Autodesk Inventor part; units mm, degrees
ref_plane "Work Plane2" through (-220.8757, 0, -44.2597) normal (-0.9238795, 0, -0.3826834) x (0, 1, 0)
ref_plane "Work Plane4" through (-216.1663, 15, -57.9216) normal (0.9238795, 0, 0.3826834) x (0, -1, 0)
ref_plane "YZ Plane" through (0, 0, 0) normal (1, 0, 0) x (0, 1, 0)
sketch "Sketch1" plane through (0, 0, 0) normal (0, 1, 0) x (-1, 0, 0)
  circle A0 centre (0, 0) radius 217.5
  circle A1 centre (0, 0) radius 312.5
  line L0 (0, 0) -> (220.9709, -220.9709)
  line L1 (0, 0) -> (312.5, 0) construction
  line L2 (312.1398, -15) -> (216.9821, -15)
  line L3 (231.3228, -210.1096) -> (164.0361, -142.8229)
  circle A2 centre (0, 0) radius 240
  circle A3 centre (0, 0) radius 290
  line L4 (285.6571, -50) -> (234.7339, -50)
  line L5 (237.3454, -166.6348) -> (201.3373, -130.6266)
  dimension "d0" = 435
  dimension "d1" = 625
  dimension "d2" = 45
  dimension "d3" = 15
  dimension "d4" = 15
  dimension "d5" = 22.5
  dimension "d6" = 22.5
  dimension "d7" = 35
  dimension "d8" = 35
extrude "Extrusion1" add sketch "Sketch1" along normal blind 10 contours A2 L4 A3 L5
sketch "Sketch2" plane through (0, 10, 0) normal (0, 1, 0) x (1, 0, 0)
  arc A0 (-237.3454, 166.6348) -> (-285.6571, 50) centre (0, 0) ccw
  line L0 (-285.6571, 50) -> (-234.7339, 50)
  arc A1 (-201.3373, 130.6266) -> (-234.7339, 50) centre (0, 0) ccw
  line L1 (-201.3373, 130.6266) -> (-237.3454, 166.6348)
  circle A2 centre (0, 0) radius 245
  circle A3 centre (0, 0) radius 285
  line L2 (-279.6426, 55) -> (-238.7467, 55)
  line L3 (-236.6281, 158.8463) -> (-207.7103, 129.9286)
  line L4 (-239.8437, 50) -> (-280.5798, 50)
  line L5 (-204.9504, 134.2398) -> (-233.7552, 163.0445)
  dimension "d11" = 5
  dimension "d12" = 5
  dimension "d13" = 5
  dimension "d14" = 5
extrude "Extrusion2" cut sketch "Sketch2" against normal up to surface (10 mm away) contours L3 A2 L2 A3
sketch "Sketch3" plane through (0, 10, 0) normal (0, 1, 0) x (1, 0, 0)
  arc A0 (-236.6281, 158.8463) -> (-279.6426, 55) centre (0, 0) ccw
  line L0 (-236.6281, 158.8463) -> (-207.7103, 129.9286)
  arc A1 (-207.7103, 129.9286) -> (-238.7467, 55) centre (0, 0) ccw
  line L1 (-238.7467, 55) -> (-279.6426, 55)
  arc A2 (-237.3454, 166.6348) -> (-285.6571, 50) centre (0, 0) ccw
  line L2 (-285.6571, 50) -> (-234.7339, 50)
  arc A3 (-201.3373, 130.6266) -> (-234.7339, 50) centre (0, 0) ccw
  line L3 (-201.3373, 130.6266) -> (-237.3454, 166.6348)
  circle A4 centre (0, 0) radius 217.5
  circle A5 centre (0, 0) radius 312.5
  line L4 (0, 0) -> (100, 0) construction
  line L5 (0, 0) -> (-220.9709, 220.9709)
  line L6 (0, 0) -> (312.5, 0) construction
  line L7 (-312.1398, 15) -> (-216.9821, 15)
  line L8 (-164.0361, 142.8229) -> (-231.3228, 210.1096)
  line L9 (-437.5, 0) -> (437.5, 0)
  dimension "d17" = 435
  dimension "d18" = 625
  dimension "d21" = 135
  dimension "d22" = 15
  dimension "d23" = 15
extrude "Extrusion3" add sketch "Sketch3" along normal blind 5 contours L0 A1 L1 A0 | L3 A3 L2 A2 | A4 L7 A5 L8
sketch "Sketch4" plane through (0, 15, 0) normal (0, 1, 0) x (1, 0, 0)
  arc A0 (-231.3228, 210.1096) -> (-312.1398, 15) centre (0, 0) ccw
  line L0 (-312.1398, 15) -> (-216.9821, 15)
  arc A1 (-164.0361, 142.8229) -> (-216.9821, 15) centre (0, 0) ccw
  line L1 (-164.0361, 142.8229) -> (-231.3228, 210.1096)
  circle A2 centre (0, 0) radius 217.5
  circle A3 centre (0, 0) radius 312.5
  line L2 (0, 0) -> (4.6194, -1.9134) construction
  line L3 (0, 0) -> (5, 0) construction
  circle A4 centre (4.6194, -1.9134) radius 242.5
  circle A5 centre (4.6194, -1.9134) radius 297.5
  line L4 (0, 0) -> (-288.7124, 119.5886) construction
  line L5 (0, 0) -> (-270.6329, 156.25)
  line L6 (0, 0) -> (-301.8518, 80.881)
  circle A6 centre (4.6194, -1.9134) radius 228.75
  circle A7 centre (4.6194, -1.9134) radius 311.25
  point P0 (-253.3489, 146.271)
  point P1 (-217.3642, 196.151)
  point P2 (-282.5739, 75.7155)
  point P3 (-292.3994, 15)
  point P4 (-205.7173, 118.7709)
  point P5 (-188.3605, 108.75)
  point P6 (-178.396, 157.1828)
  point P7 (-210.0889, 56.2931)
  point P8 (-229.4479, 61.4804)
  point P9 (-237.2901, 15)
  point P10 (-295.8554, 79.2742)
  point P11 (-265.2567, 153.146)
  point P12 (-193.8094, 111.8959)
  point P13 (-216.1663, 57.9216)
  dimension "d26" = 625
  dimension "d27" = 435
  dimension "d28" = 5
  dimension "d29" = 22.5
  dimension "d30" = 485
  dimension "d31" = 595
  dimension "d33" = 15
  dimension "d36" = 457.5
  dimension "d37" = 622.5
extrude "Extrusion4" cut sketch "Sketch4" against normal blind 10 contours L1 A7 L5 A0 | L5 A7 L6 A0 | L1 A5 L5 A7 | L6 A7 L0 A0 | L6 A5 L0 A7 | L1 A6 L5 A4 | L1 A1 L5 A6 | L6 A6 L0 A4 | L5 A1 L6 A6 | L6 A1 L0 A6
sketch "Sketch5" plane through (0, 15, 0) normal (0, 1, 0) x (1, 0, 0)
  arc A0 (-282.5739, 75.7155) -> (-292.3994, 15) centre (4.6194, -1.9134) ccw
  line L0 (-292.3994, 15) -> (-237.2901, 15)
  arc A1 (-229.4479, 61.4804) -> (-237.2901, 15) centre (4.6194, -1.9134) ccw
  line L1 (-229.4479, 61.4804) -> (-216.1663, 57.9216)
  arc A2 (-193.8094, 111.8959) -> (-216.1663, 57.9216) centre (4.6194, -1.9134) ccw
  line L2 (-193.8094, 111.8959) -> (-205.7173, 118.7709)
  arc A3 (-178.396, 157.1828) -> (-205.7173, 118.7709) centre (4.6194, -1.9134) ccw
  line L3 (-178.396, 157.1828) -> (-217.3642, 196.151)
  arc A4 (-217.3642, 196.151) -> (-253.3489, 146.271) centre (4.6194, -1.9134) ccw
  line L4 (-253.3489, 146.271) -> (-265.2567, 153.146)
  arc A5 (-265.2567, 153.146) -> (-295.8554, 79.2742) centre (4.6194, -1.9134) ccw
  line L5 (-295.8554, 79.2742) -> (-282.5739, 75.7155)
  arc A6 (-157.7572, 146.5246) -> (-215.1597, 7.9427) centre (4.6194, -1.9134) ccw
  arc A7 (-254.0861, 186.4253) -> (-311.4886, 47.8434) centre (4.6194, -1.9134) ccw
  line L6 (-311.4886, 47.8434) -> (-215.1597, 7.9427)
  line L7 (-157.7572, 146.5246) -> (-254.0861, 186.4253)
  line L8 (-291.0221, 120.5453) -> (-198.6341, 82.2769) construction
  line L9 (-282.9381, 117.1968) -> (-206.718, 85.6254) construction
  point P0 (0, 0)
  point P1 (-244.8281, 101.4111)
  point P2 (-244.8281, 101.4111)
  point P3 (-232.656, 177.5487)
  point P4 (-179.7358, 155.6284)
  point P5 (-237.1383, 17.0465)
  point P6 (-290.0585, 38.9667)
  dimension "d38" = 150
  dimension "d39" = 104.2656
extrude "Extrusion5" cut sketch "Sketch5" against normal blind 10 contours L6 A1 L0 A0 | A4 L3 A3 L7
ref_plane "Work Plane2" through (-220.8757, 0, -44.2597) normal (-0.9238795, 0, -0.3826834) x (0, 1, 0)
ref_plane "Work Plane1" through (-234.7339, 0, -50) normal (-0.9238795, 0, -0.3826834) x (0, 1, 0)
sketch "Sketch7" plane through (0, 10, 0) normal (0, -1, 0) x (1, 0, 0)
  arc A0 (-279.6426, -55) -> (-236.6281, -158.8463) centre (0, 0) ccw
  line L0 (-236.6281, -158.8463) -> (-207.7103, -129.9286)
  arc A1 (-238.7467, -55) -> (-207.7103, -129.9286) centre (0, 0) ccw
  arc A2 (-238.7467, -55) -> (-207.7103, -129.9286) centre (0, 0) ccw
  line L1 (-238.7467, -55) -> (-279.6426, -55)
  arc A3 (-279.6426, -55) -> (-236.6281, -158.8463) centre (0, 0) ccw
  arc A4 (-291.5761, -93.715) -> (-272.4419, -139.9089) centre (4.6194, 1.9134) ccw
  line L2 (-195.885, -108.198) -> (-272.4419, -139.9089)
  arc A5 (-215.0192, -62.0041) -> (-195.885, -108.198) centre (4.6194, 1.9134) ccw
  line L3 (-215.0192, -62.0041) -> (-291.5761, -93.715)
  arc A6 (-279.6426, -55) -> (-236.6281, -158.8463) centre (0, 0) ccw
  line L4 (-279.6426, -55) -> (-238.7467, -55)
  arc A7 (-238.7467, -55) -> (-207.7103, -129.9286) centre (0, 0) ccw
  line L5 (-207.7103, -129.9286) -> (-236.6281, -158.8463)
  arc A8 (-285.6571, -50) -> (-237.3454, -166.6348) centre (0, 0) ccw
  line L6 (-201.3373, -130.6266) -> (-237.3454, -166.6348)
  arc A9 (-234.7339, -50) -> (-201.3373, -130.6266) centre (0, 0) ccw
  line L7 (-285.6571, -50) -> (-234.7339, -50)
  line L8 (-233.2223, -155.4405) -> (-236.0507, -152.6121) construction
  line L9 (-236.0507, -152.6121) -> (-238.8791, -155.4405) construction
  line L10 (-209.8621, -132.0804) -> (-212.6905, -129.2519) construction
  line L11 (-212.6905, -129.2519) -> (-209.8621, -126.4235) construction
  circle A10 centre (-212.6905, -129.2519) radius 1.75
  circle A11 centre (-236.0507, -152.6121) radius 1.75
  line L12 (-274.8261, -55) -> (-274.8261, -59) construction
  line L13 (-274.8261, -59) -> (-278.8261, -59) construction
  line L14 (-241.7898, -55) -> (-241.7898, -59) construction
  line L15 (-241.7898, -59) -> (-237.7898, -59) construction
  circle A12 centre (-241.7898, -59) radius 1.75
  circle A13 centre (-274.8261, -59) radius 1.75
  line L16 (-233.2223, -162.5116) -> (-226.8583, -156.1476)
  line L17 (-226.8583, -156.1476) -> (-236.0507, -146.9553)
  line L18 (-236.0507, -146.9553) -> (-242.4147, -153.3192)
  line L19 (-242.4147, -153.3192) -> (-233.2223, -162.5116)
  line L20 (-209.155, -138.4443) -> (-201.3373, -130.6266)
  line L21 (-201.3373, -130.6266) -> (-210.5297, -121.4342)
  line L22 (-210.5297, -121.4342) -> (-218.3474, -129.2519)
  line L23 (-218.3474, -129.2519) -> (-209.155, -138.4443)
  line L24 (-285.6571, -50) -> (-270.8261, -50)
  line L25 (-270.8261, -50) -> (-270.8261, -63)
  line L26 (-270.8261, -63) -> (-285.6571, -63)
  line L27 (-285.6571, -63) -> (-285.6571, -50)
  line L28 (-234.7339, -50) -> (-245.7898, -50)
  line L29 (-245.7898, -50) -> (-245.7898, -63)
  line L30 (-245.7898, -63) -> (-234.7339, -63)
  line L31 (-234.7339, -63) -> (-234.7339, -50)
  line L32 (-236.6281, -158.8463) -> (-207.7103, -129.9286)
  line L33 (-238.7467, -55) -> (-279.6426, -55)
  arc A14 (-279.6426, -55) -> (-236.6281, -158.8463) centre (0, 0) ccw
  line L34 (-236.6281, -158.8463) -> (-207.7103, -129.9286)
  arc A15 (-238.7467, -55) -> (-207.7103, -129.9286) centre (0, 0) ccw
  line L35 (-238.7467, -55) -> (-279.6426, -55)
  point P0 (-214.4385, -125.3431)
  point P1 (-277.9496, -63)
  point P2 (-270.8261, -55)
  point P3 (-236.7615, -63)
  point P4 (-245.7898, -55)
  point P5 (-212.6905, -134.9088)
  point P6 (-211.9634, -122.8679)
  point P7 (-241.0878, -151.9923)
  point P8 (-230.3939, -152.6121)
  dimension "d51" = 4
  dimension "d52" = 4
  dimension "d54" = 4
  dimension "d55" = 4
  dimension "d56" = 3.5
  dimension "d57" = 3.5
  dimension "d58" = 4
  dimension "d59" = 4
  dimension "d60" = 4
  dimension "d61" = 4
  dimension "d62" = 3.5
  dimension "d63" = 3.5
  dimension "d64" = 4
  dimension "d65" = 4
  dimension "d66" = 5
  dimension "d71" = 4
  dimension "d72" = 4
  dimension "d73" = 4
  dimension "d74" = 4
  dimension "d75" = 4
  dimension "d76" = 4
extrude "Extrusion7" add sketch "Sketch7" along normal blind 10 contours L1 L25 L26 A0 | L1 A1 L30 L29 | L18 L17 L0 A0 | A1 L0 L23 L22
extrude "Extrusion8" cut sketch "Sketch7" against normal up to next contours A10 | A11 | A12 | A13
ref_plane "Work Plane4" through (-216.1663, 15, -57.9216) normal (0.9238795, 0, 0.3826834) x (0, -1, 0)
sketch "Sketch9" plane through (-216.1663, 15, -57.9216) normal (0.9238795, 0, 0.3826834) x (0, -1, 0)
  line L0 (5, 58.4214) -> (5, 0)
  line L1 (0, 58.4214) -> (5, 58.4214)
  line L2 (0, 0) -> (0, 58.4214)
  line L3 (0, 0) -> (5, 0)
  line L4 (15, -14.4241) -> (15, 72.8455)
  line L5 (15, 72.8455) -> (5, 72.8455)
  line L6 (5, -14.4241) -> (5, 72.8455)
  line L7 (15, -14.4241) -> (5, -14.4241)
  line L8 (-2, 5.2107) -> (2, 5.2107)
  line L9 (2, 5.2107) -> (2, 53.2107)
  line L10 (2, 53.2107) -> (-2, 53.2107)
  line L11 (-2, 53.2107) -> (-2, 5.2107)
  line L12 (-2, 5.2107) -> (2, 53.2107) construction
  line L13 (2, 5.2107) -> (-2, 53.2107) construction
  point P0 (15, 29.2107)
  point P1 (0, 29.2107)
  dimension "d85" = 4
  dimension "d86" = 48
extrude "Extrusion10" cut sketch "Sketch9" against normal up to next contours L10 L9 L8 L2 | L2 L8 L11 L10
sketch "Sketch10" plane through (0, 10, 0) normal (0, -1, 0) x (1, 0, 0)
  arc A0 (-291.2664, -94.6691) -> (-272.8976, -139.0153) centre (4.6194, 1.9134) ccw
  line L0 (-214.736, -62.9692) -> (-291.2664, -94.6691)
  arc A1 (-214.736, -62.9692) -> (-196.3672, -107.3154) centre (4.6194, 1.9134) ccw
  line L1 (-196.3672, -107.3154) -> (-272.8976, -139.0153)
  line L2 (-245.7898, -63) -> (-245.7898, -55)
  line L3 (-245.7898, -55) -> (-270.8261, -55)
  line L4 (-270.8261, -55) -> (-270.8261, -63)
  line L5 (-270.8261, -63) -> (-277.9496, -63)
  arc A2 (-277.9496, -63) -> (-241.0878, -151.9923) centre (0, 0) ccw
  line L6 (-241.0878, -151.9923) -> (-236.0507, -146.9553)
  line L7 (-236.0507, -146.9553) -> (-230.3939, -152.6121)
  line L8 (-230.3939, -152.6121) -> (-212.6905, -134.9088)
  line L9 (-212.6905, -134.9088) -> (-218.3474, -129.2519)
  line L10 (-218.3474, -129.2519) -> (-211.9634, -122.8679)
  arc A3 (-236.7615, -63) -> (-211.9634, -122.8679) centre (0, 0) ccw
  line L11 (-236.7615, -63) -> (-245.7898, -63)
  point P0 (-216.0774, -115.4796)
  point P1 (-234.4462, -71.1334)
  point P2 (-271.5548, -86.5043)
  point P3 (-253.186, -130.8505)
extrude "Extrusion11" cut sketch "Sketch10" against normal blind 10 contours L0 A3 L1 A2
properties part number "Battery Module Third Iteration Top wING" material "PLA Plastic"
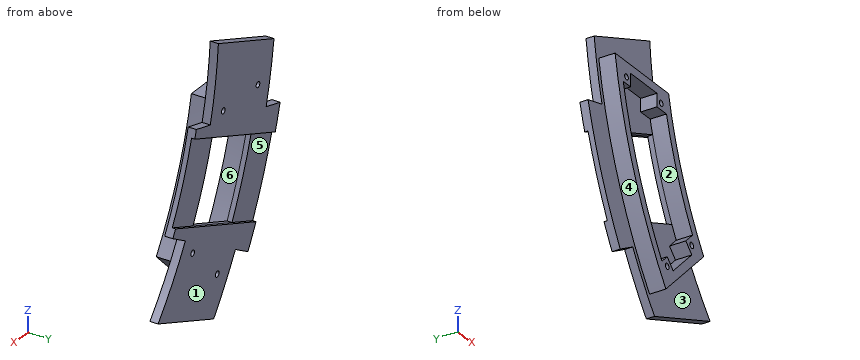
Geometry: final body of the model. Coordinates: model frame, mm. Face numbers are marked on the shaded views. A direction names the side the tool comes from. Give positions to 0.01 mm unless a question says otherwise; leave off trailing zeros. Write each loop counter-clockwise with the first axis right and the second up, starting at its lowest first coordinate (ties: lowest second). Pieces come first, ordered by that corner, then holes. Notation, with made-up numbers: (-21, 4.5) -> (15, 4.5) arc R17 cw to (15, 19.5) -> close; hole circle Ø6 at (51.5, 15.5). An arc over 180 degrees is marked (long way). Answer in a Markdown table with one row per item.
(1) Section query C-C on z = -69. Return loops of the section in (x, y), then the cut area to 3 significant figures.
Answers below:
| item | result |
|---|---|
| outline | (-284.31, 10) -> (-281.67, 10) -> (-281.67, 0) -> (-276.52, 0) -> (-276.52, 10) -> (-235.08, 10) -> (-235.08, 0) -> (-229.87, 0) -> (-229.87, 10) -> (-212.86, 10) -> (-212.86, 13) -> (-229.3, 13) -> (-229.3, 15) -> (-284.31, 15) -> close |
| area | 428 mm^2 |
(2) Set-up query: the marked faces 1 and 2. Return all of +Z, -Z, +X, -X, +Y, -Y with unobstructed straight access to the full face (end or side cutting, diameter ignored); none if empty.
Answers below:
| item | result |
|---|---|
| face 1 | +Z, -Z, +X, -X, +Y |
| face 2 | -Y |
(3) Pin query (flat end, axial travel): pin 1 (4 mm diameter, centred on y = 1.5, z = -118.5, fed in from +X); pin 2 (3 mm diameter, centred on x = -244.5, z = -74, fed in from -Y); pin 3 (2 mm diameter, centred on x = -274.83, z = -59, fed in from +Y); pin 4 (3 mm diameter, centred on x = -257, y = 2.5, fed in from -Z). Return the tip coordinate at first contact, or that it passes through.
Answers below:
| item | result |
|---|---|
| pin 1 | x = -207.56 |
| pin 2 | y = 10 |
| pin 3 | through |
| pin 4 | z = -137.19 |
(4) Section query D-D on x = -247.5. Return loops of the section in (y, z).
Answers below:
| item | result |
|---|---|
| outline | (0, -151.14) -> (10, -151.14) -> (10, -156.02) -> (15, -156.02) -> (15, -128.5) -> (10, -128.5) -> (10, -141.31) -> (0, -141.31) -> close; (0, -55) -> (10, -55) -> (10, -76.54) -> (15, -76.54) -> (15, -21.34) -> (10, -21.34) -> (10, -50) -> (0, -50) -> close |
(5) Section query B-B on y = 3.25. Return loops of the section in (x, z).
Answers below:
| item | result |
|---|---|
| outline | (-285.66, -50) arc R290 ccw to (-237.35, -166.63) -> (-201.34, -130.63) arc R240 cw to (-234.73, -50) -> close; hole (-277.95, -63) arc R285 ccw to (-241.09, -151.99) -> (-236.05, -146.96) -> (-230.39, -152.61) -> (-212.69, -134.91) -> (-218.35, -129.25) -> (-211.96, -122.87) arc R245 cw to (-236.76, -63) -> (-245.79, -63) -> (-245.79, -55) -> (-270.83, -55) -> (-270.83, -63) -> close; hole circle Ø3.5 at (-274.83, -59); hole circle Ø3.5 at (-241.79, -59); hole circle Ø3.5 at (-236.05, -152.61); hole circle Ø3.5 at (-212.69, -129.25) |
(6) Draft query along Z for the marked faces 3, 4, 5 and 6. Return one class per face: +Z half, -Z half, draft (parallel to the pull), parting line (faces both ways), or undercut.
Answers below:
| item | result |
|---|---|
| face 3 | draft |
| face 4 | -Z half |
| face 5 | undercut |
| face 6 | undercut |
(7) Ray query, line 1 along Y through (x, z) = (-269, -118.5); line 2 along Z through (x, y) = (-250, 7.75); line 3 along X through (y, z) = (1, -61). Return the intervals inside material, ascending. Write a range as [from, to].
Answers below:
| item | result |
|---|---|
| line 1 | [10, 13] |
| line 2 | [-146.97, -136.84], [-55, -50] |
| line 3 | [-283.51, -270.83], [-245.79, -232.12] |
(8) Section query A-A on x = -225. Return loops of the section in (y, z), then the cut area to 3 significant figures.
Answers below:
| item | result |
|---|---|
| outline | (0, -154.29) -> (10, -154.29) -> (10, -174.38) -> (15, -174.38) -> (15, -119.18) -> (10, -119.18) -> (10, -147.22) -> (0, -147.22) -> close; (0, -96.95) -> (13, -96.95) -> (13, -67.22) -> (15, -67.22) -> (15, -60.29) -> (10, -60.29) -> (10, -83.52) -> (0, -83.52) -> close |
| area | 605 mm^2 |
